Can you work these out from the model? Positions are in its coordinate system, mm. Face numbers are marked on the shaded views. A direction names the side the tool comes from. Coordinates: 2 decimals unless noted, no trailing zeros. Order: outer loops, then holes, each group sorted by start corner. A loop starts at its lowest first (then second) coordinate and runs counter-clockwise, first axis right, second up. Notation, with made-up numbers: (-36, 14.5) -> (-11, 14.5) arc R23 cw to (-11, 37.5) -> close; hole circle Ø7 at (-7.5, 26). An arc over 180 degrees is marked (long way). Answer as a JSON object with one key per item and string values. Group by question number.
(1) I want a section at C-C, the plane x = 15. List the corners of the cut face in (y, z) for me, plus the area to 3 significant figures.
(2) I want a section at A-A, the plane z = 12.5. List the corners of the cut face in (x, y) for me, plus the area to 3 significant figures.
(3) I want a section at B-B, the plane y = 89. List the corners of the cut face in (x, z) for me.
(4) If we mould it in two halves opening along Y, with no side actions, what happens to the marked faces 1, 2 and 3? For each: pulls with the +Y half, pulls with the -Y half, needs draft (parallel to the pull), parting line crosses it, or undercut.
(5) For pin 1 (2 mm diameter, centred on x = -22.5, y = 68.5, fed in from +Z); pin 2 (5 mm diameter, centred on y = 13.5, z = 36.5, fed in from +X); pin 3 (0.8 mm diameter, centred on x = -20, z = 50.5, fed in from -Y), each with a flat end and sliding along its axis, tell me the tip position at first contact or that it passes through.
(6) I need wall thicknesses on line 1 (Y direction, x = 6, z = -34); line 2 (Y direction, x = 33, z = -41); line 3 (Y direction, x = -45, z = 40.5). Which ranges of each line are inside material? Lowest first, please.
(7) Which directions (+Z, -Z, +X, -X, +Y, -Y) give clear straight access to the entire face, cutting with the end or side of a thin tool? Please do the marked faces 4, 5 and 6.
(8) I want a section at D-D, the plane x = -35. List the corners of the cut face in (y, z) for me, plus the area to 3 significant figures.
from build123d import *

# Parameters (mm, degrees)
EXTRUDE_1_DEPTH     = 50
EXTRUDE_1_2_DEPTH   = 50
SKETCH_3_W          = 80
SKETCH_3_H          = 70
EXTRUDE_2_DEPTH     = 1
SKETCH_4_R          = 3
SKETCH_4_R_2        = 6
SKETCH_4_R_3        = 10
CUT_EXTRUDE_1_DEPTH = 10
SKETCH_5_R          = 7.5
SKETCH_5_R_2        = 5
EXTRUDE_3_DEPTH     = 20
SKETCH_6_R          = 2
EXTRUDE_4_DEPTH     = 16


with BuildPart() as part:
    # 草图1 → Extrude 1 (new, symmetric)
    with BuildSketch(Plane.XY):
        Polygon((-50, 10.796505179), (50, 10.796505179), (60, -9.203494821), (-60, -9.203494821), align=None)
        Polygon((-48.763932023, 8.796505179), (48.763932023, 8.796505179), (56.763932023, -7.203494821), (-56.763932023, -7.203494821), align=None, mode=Mode.SUBTRACT)
    extrude(amount=EXTRUDE_1_DEPTH, both=True)

    # 草图2 → Extrude 1 2 (add, symmetric)
    with BuildSketch(Plane.XY):
        with BuildLine():
            Line((50, 26.346525195), (50, 126.346525195))
            Line((50, 126.346525195), (-50, 126.346525195))
            Line((-50, 126.346525195), (-50, 26.346525195))
            ThreePointArc((-50, 26.346525195), (0, 8.796505179), (50, 26.346525195))
        make_face()
    extrude(amount=EXTRUDE_1_2_DEPTH, both=True)

    # 草图3 → 凸台-拉伸2 (add)
    with BuildSketch(Plane.XY.offset(50)):
        with Locations((0, 71.346525195)):
            Rectangle(SKETCH_3_W, SKETCH_3_H)
    extrude(amount=EXTRUDE_2_DEPTH)

    # 草图4 → 切除-拉伸1 (cut)
    with BuildSketch(Plane.XY.offset(50)):
        with Locations((-35, 116.346525195)):
            Circle(SKETCH_4_R)
        with Locations((-5, 116.346525195)):
            Circle(SKETCH_4_R_2)
        with Locations((30, 116.346525195)):
            Circle(SKETCH_4_R_2)
        with Locations((0, 23.796505179)):
            Circle(SKETCH_4_R_3)
    extrude(amount=-CUT_EXTRUDE_1_DEPTH, mode=Mode.SUBTRACT)

    # 草图5 → 凸台-拉伸3 (add)
    with BuildSketch(Plane.XY.offset(40)):
        with Locations((0, 23.796505179)):
            Circle(SKETCH_5_R)
        with Locations((-5, 116.346525195)):
            Circle(SKETCH_5_R_2)
        with Locations((30, 116.346525195)):
            Circle(SKETCH_5_R_2)
    extrude(amount=EXTRUDE_3_DEPTH)

    # 草图6 → 凸台-拉伸4 (add)
    with BuildSketch(Plane.XY.offset(40)):
        with Locations((-35, 116.346525195)):
            Circle(SKETCH_6_R)
    extrude(amount=EXTRUDE_4_DEPTH)


solid = part.part
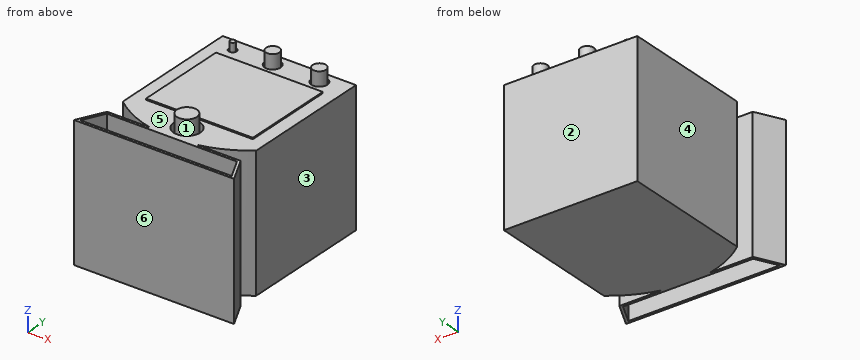
Computed values:
{
 "1": {"outline": "(-9.2, -50) -> (-7.2, -50) -> (-7.2, 50) -> (-9.2, 50) -> close; (8.8, -50) -> (126.35, -50) -> (126.35, 50) -> (106.35, 50) -> (106.35, 51) -> (36.35, 51) -> (36.35, 50) -> (8.8, 50) -> close", "area": "12,000 mm2"},
 "2": {"outline": "(-60, -9.2) -> (60, -9.2) -> (50, 10.8) -> (17.78, 10.8) arc R80 ccw to (50, 26.35) -> (50, 126.35) -> (-50, 126.35) -> (-50, 26.35) arc R80 ccw to (-17.78, 10.8) -> (-50, 10.8) -> close; hole (-56.76, -7.2) -> (56.76, -7.2) -> (48.76, 8.8) -> (-48.76, 8.8) -> close", "area": "11,700 mm2"},
 "3": {"outline": "(-50, -50) -> (50, -50) -> (50, 50) -> (40, 50) -> (40, 51) -> (-40, 51) -> (-40, 50) -> (-50, 50) -> close"},
 "4": {"face 1": "undercut", "face 2": "pulls with the +Y half", "face 3": "needs draft"},
 "5": {"pin 1": "stops at z = 51", "pin 2": "stops at x = 33.18", "pin 3": "stops at y = 36.35"},
 "6": {"line 1": "y = -9.2 to -7.2, 8.8 to 126.35", "line 2": "y = -9.2 to -7.2, 8.8 to 10.8, 15.92 to 126.35", "line 3": "y = -9.2 to -7.2, 8.8 to 10.8, 22.65 to 126.35"},
 "7": {"face 4": "+Z, -Z, -X, +Y", "face 5": "+Z", "face 6": "+Z, -Z, +X, -X, -Y"},
 "8": {"outline": "(-9.2, -50) -> (-7.2, -50) -> (-7.2, 50) -> (-9.2, 50) -> close; (8.8, -50) -> (10.8, -50) -> (10.8, 50) -> (8.8, 50) -> close; (16.86, -50) -> (126.35, -50) -> (126.35, 50) -> (119.35, 50) -> (119.35, 40) -> (118.35, 40) -> (118.35, 56) -> (114.35, 56) -> (114.35, 40) -> (113.35, 40) -> (113.35, 50) -> (106.35, 50) -> (106.35, 51) -> (36.35, 51) -> (36.35, 50) -> (16.86, 50) -> close", "area": "11,400 mm2"}
}
